The listing builds one solid part. Answer for the finished solid, in the listing's coordinates (mm). A direction names the side the tool comes from. Round coordinates to 2 decimals unless told otherwise and drop trailing zeros. Write each loop counter-clockwise with the first axis right and the second up, starting at its lowest first coordinate (ties: lowest second). Pieces come first, ordered by that corner, then holes.
Item 1: Find the intervals of material crossed by probe 1 along Y at (x, z) = (-78, 38.5); probe 2 along X at (y, z) = (-184, 44); probe 3 along Z at (x, y) = (-60, -116), in increasing order.
Item 2: Find section B-B on z = 65. Give the vertices of the cut face in (x, y), then the cut area to 3 significant figures.
Item 3: A tool of negligible diameter and unlimited length cuts with its end or side. For faces 1 (the face through (-81.56, -150.27, 14.87)), 2 (the face through (-77.61, 4.83, 40.23)), 3 (the face through (-79.716, -314.192, 41.999)), from which of +Z, -Z, +X, -X, +Y, -Y can it reach the whole face along a straight path? Write none if from no direction.
Item 4: Each of these flat-tipped pins is pushed along its axis until it touches: pin 1 (6 mm diameter, centred on x = -63, z = 49, fed in from +Y); pin 2 (10 mm diameter, centred on y = -239, z = 59.5, fed in from +X); pin 3 (8 mm diameter, centred on x = -88, y = -189.5, fed in from +Z); pin 4 (5 mm diameter, centred on y = -209.5, z = 46.5, fed in from -X). Where does it stop, or does it pass through?
Item 5: Find section C-C on y = -255.5. Give the vertices of the cut face in (x, z).
Item 6: Find section D-D on z = 34. Give the vertices of the cut face in (x, y), then the cut area to 3 significant figures.
Item 7: Find section A-A on x = -72. Give the vertices of the cut face in (y, z) (3 decimals), then the cut area to 3 significant figures.
```python
from build123d import *

# Parameters (mm, degrees)
F0_R     = 31.75
F1_DEPTH = 304.8
F2_R     = 6.35
F3_DEPTH = 9.525
F4_R     = 6.35
F5_DEPTH = 19.05


with BuildPart() as f1:
    # F0 (on Front) → F1 (new body)
    with BuildSketch(Plane.XZ):
        with Locations((-74.6771916747, 45.8630174398)):
            Circle(F0_R)
    extrude(amount=F1_DEPTH)

    # F2 (on face) → F3 (join, symmetric)
    with BuildSketch(Plane(origin=(0, 0, 0), x_dir=(-1, 0, 0), z_dir=(0, 1, 0))):
        with Locations((74.6771916747, 45.8630174398)):
            Circle(F2_R)
    extrude(amount=F3_DEPTH, both=True)

    # F4 (on face) → F5 (join)
    with BuildSketch(Plane.XZ.offset(304.8)):
        with Locations((-74.6771916747, 45.8630174398)):
            Circle(F4_R)
    extrude(amount=F5_DEPTH)


solid = f1.part
```
Check values:
1. probe 1: y = -304.8 to 0
1. probe 2: x = -106.37 to -42.98
1. probe 3: z = 17.71 to 74.02
2. outline: (-100.01, -304.8) - (-49.34, -304.8) - (-49.34, 0) - (-100.01, 0) - close
2. area: 15,400 mm2
3. face 1: +Y, -Y
3. face 2: +Y
3. face 3: -Y
4. pin 1: stops at y = 0
4. pin 2: stops at x = -44.12
4. pin 3: stops at z = 76.21
4. pin 4: stops at x = -106.43
5. outline: circle Ø63.5 at (-74.68, 45.86)
6. outline: (-104.13, -304.8) - (-45.23, -304.8) - (-45.23, 0) - (-104.13, 0) - close
6. area: 18,000 mm2
7. outline: (-323.85, 40.105) - (-304.8, 40.105) - (-304.8, 14.226) - (0, 14.226) - (0, 40.105) - (9.525, 40.105) - (9.525, 51.621) - (0, 51.621) - (0, 77.5) - (-304.8, 77.5) - (-304.8, 51.621) - (-323.85, 51.621) - close
7. area: 19,600 mm2
